Autodesk Inventor part; units mm, degrees
ref_plane "Work Plane1" through (0, 20, 0) normal (0, 1, 0) x (-1, 0, 0)
ref_plane "YZ Plane" through (0, 0, 0) normal (1, 0, 0) x (0, 1, 0)
ref_plane "XY Plane" through (0, 0, 0) normal (0, 0, 1) x (1, 0, 0)
sketch "Sketch1" plane through (0, 0, 0) normal (0, 0, 1) x (1, 0, 0)
  line L0 (0, 0) -> (0, 20)
  line L1 (0, 0) -> (20, 0)
  arc A0 (20, 0) -> (0, 20) centre (0, 0) ccw
  line L2 (0, -4.828427) -> (0, 28.970563)
  dimension "d2" = 20
sketch "Sketch1 outline for Revolution1" plane through (0, 0, 0) normal (0, 0, 1) x (1, 0, 0)
  line L0 (0, 0) -> (0, 20)
  arc A0 (0, 20) -> (20, 0) centre (0, 0) cw
  line L1 (20, 0) -> (0, 0)
revolve "Revolution1" add sketch "Sketch1 outline for Revolution1" angle 360 about axis through (0, -10, 0) along (0, 1, 0)
ref_plane "Work Plane1" through (0, 20, 0) normal (0, 1, 0) x (-1, 0, 0)
sketch "Sketch2" plane through (0, 20, 0) normal (0, 1, 0) x (-1, 0, 0)
  point P0 (0, 0)
  point P1 (0, 0)
hole "Hole1" at (0, 20, 0) direction (0, -1, 0) diameter 4.5 end through all counterbore diameter 8 counterbore depth 4
shell "Shell1" thickness 5 removed faces 1 at (13.884144, 0, 1.68584)
sketch "Sketch3" plane through (0, 0, 0) normal (0, -1, 0) x (1, 0, 0)
  circle A0 centre (0, 0) radius 7.25
  circle A1 centre (0, 0) radius 2.25
sketch "Sketch3 outline for Extrusion1" plane through (0, 0, 0) normal (0, -1, 0) x (1, 0, 0)
  circle A0 centre (0, 0) radius 7.25
  circle A1 centre (0, 0) radius 2.25
extrude "Extrusion1" cut sketch "Sketch3 outline for Extrusion1" against normal up to surface (11 mm away)
properties part number "Ball_Upper Half" material "Nylon 6/6"
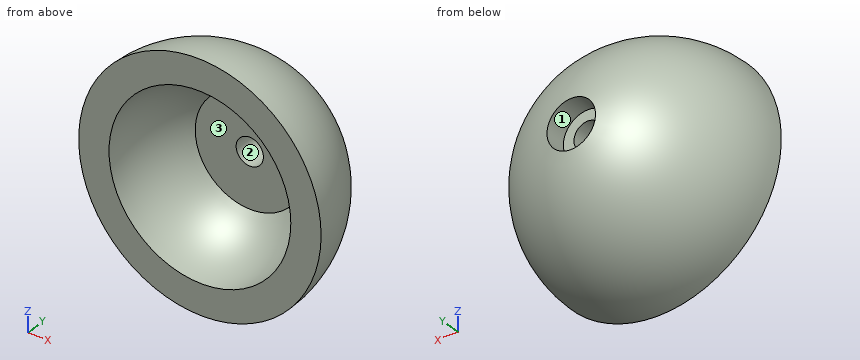
Work out the finished part from the listing and answer in its coordinate system (mm). Face numbers are marked on the shaded views. A direction names the side the tool comes from. Coordinates: 2 decimals unless noted, no trailing zeros. Write each loop counter-clockwise with the first axis right and the second up, starting at its lowest first coordinate (ties: lowest second). Pieces come first, ordered by that corner, then holes. Notation, with made-up numbers: M 34.5,14.5 L 52.5,14.5 A25 ccw 52.5,35.5 Z; hole C 0,24.25 d3. An arc over 180 degrees is marked long. Answer as CSV lines item,"result". Start each with the question number.
Item 1: Section A-A on z = 0 is taken. Write down the section's boundary in (x, y).
Item 2: A tool of negligible diameter and unlimited length cuts with its end or side. For the marked faces 1, 2 and 3, from which of +Z, -Z, +X, -X, +Y, -Y can it reach the whole face along a straight path? Write none if from no direction.
Item 3: Consider L1, parallel to Z at x = -3.5, y = 12.75; L2, parallel to X at y = 18.55, z = 0; L3, parallel to Z at x = 0, y = 17.5. Determine where each line is inside the solid, lowest interval first.
Item 4: Section B-B on x = 1 is taken. Write down the section's boundary in (y, z), and give its area (3 significant figures).
Item 5: Section D-D on y = 8 is taken. Write down the section's boundary in (x, z).
Item 6: Section C-C on z = -12 is taken. Write down the section's boundary in (x, y), and give its area (3 significant figures).
Item 7: Flat-ended cylindrical pins translate along their axes: P1, Ø5.5, axis at x = 0, z = 4, coming from the -Y side; P2, Ø2, axis at x = -9, z = -12.5, coming from the +Y side; P3, Ø6, axis at y = 17.5, z = 0.5, coming from the +X side. Find the tip coordinate at first contact, or state that the pin passes through.
Checks:
1,outline,"M -20,0 L -15,0 A15 cw -9,12 L -9,11 L -2.25,11 L -2.25,16 L -4,16 L -4,19.6 A20 ccw Z; M 2.25,11 L 9,11 L 9,12 A15 cw 15,0 L 20,0 A20 ccw 4,19.6 L 4,16 L 2.25,16 Z"
2,face 1,"+Y"
2,face 2,"+Y, -Y"
2,face 3,"-Y"
3,L1,"z = -15.01 to 15.01"
3,L2,"x = -7.48 to -4, 4 to 7.48"
3,L3,"z = -9.68 to -4, 4 to 9.68"
4,outline,"M 0,-19.97 A19.97 ccw 19.6,-3.87 L 16,-3.87 L 16,-2.02 L 11,-2.02 L 11,-8.94 L 12,-8.94 A14.97 cw 0,-14.97 Z; M 0,14.97 A14.97 cw 12,8.94 L 11,8.94 L 11,2.02 L 16,2.02 L 16,3.87 L 19.6,3.87 A19.97 ccw 0,19.97 Z"
4,area,"279 mm²"
5,outline,"C 0,0 d36.66; hole C 0,0 d25.38"
6,outline,"M -16,0 L -9,0 A9 cw 9,0 L 16,0 A16 ccw Z"
6,area,"275 mm²"
7,P1,"stops at y = 11"
7,P2,"stops at y = 13.88"
7,P3,"stops at x = 13.77"
